Autodesk Inventor part; units mm, degrees
ref_plane "YZ Plane" through (0, 0, 0) normal (1, 0, 0) x (0, 1, 0)
ref_plane "XZ Plane" through (0, 0, 0) normal (0, 1, 0) x (-1, 0, 0)
ref_plane "XY Plane" through (0, 0, 0) normal (0, 0, 1) x (1, 0, 0)
sketch "Sketch1" plane through (0, 0, 0) normal (0, 1, 0) x (-1, 0, 0)
  line L0 (-4, 0) -> (-4, 12.7)
  line L1 (-4, 12.7) -> (-5.1, 12.7)
  line L2 (-4, 0) -> (-5.1, 0)
  line L3 (-5.1, 12.7) -> (-5.1, 8.7)
  line L4 (-5.1, 8.7) -> (-4.6, 8.7)
  line L5 (-4.6, 8.7) -> (-4.6, 7.7)
  line L6 (-4.6, 7.7) -> (-5.1, 7.7)
  line L7 (-5.1, 0) -> (-5.1, 7.7)
  line L8 (-5.1, 8.7) -> (-5.1, 12.7)
  line L9 (0, -2.54) -> (0, 15.24)
  point P0 (0, 0)
  dimension "d0" = 5.1
  dimension "d1" = 12.7
  dimension "d2" = 4
  dimension "d3" = 4
  dimension "d4" = 0.5
  dimension "d5" = 1
revolve "Revolution1" add sketch "Sketch1" angle 360 about axis through (0, 0, -10) along (0, 0, 1)
thread "Thread1"
properties part number "M8-HEATINSERT"
Check sheet for the modelled part. Datum: model origin and axes. Units: mm. A direction names the side the tool comes from. Coordinates: 2 decimals unless noted, no trailing zeros. Loops run counter-clockwise (first coordinate to the right, second up) from the corner with the lowest first, then second, coordinate; pieces in that order, holes last.
1) Sectioned sample at A-A (x = 0). Record the boundary of the cut face in (y, z).
2) Release check for a two-part mould opening along Z. For faces 3 (the face through (-3, -3, 0)), 4 (the face through (-0.867, -3.905, 6.439)), 5 (the face through (-1.2, 4.6, 7.7)) record: released by +Z, released by -Z, zero draft, split by the parting line, or undercut.
3) Sectioned sample at C-C (z = 6). Record the boundary of the cut face in (x, y), and give its area (3 significant figures).
4) Sectioned sample at B-B (y = 2). Record the boundary of the cut face in (x, z).
5) Material ranges on probe 1 along Y at (x, z) = (0, 6); probe 2 along Z at (x, y) = (-3.5, 3.5); probe 3 along Y at (x, z) = (-1, 1.75), recorded low to high.
6) Access from +Z, -Z, +X, -X, +Y, -Y to the whole of each face (thin tool, end or side, straight path). Record for faces 1 (the face through (-3, -3, 12.7)), 2 (the face through (-3.65, 2.8, 8.19)).
7) Gauge pin test, flat ends, axial feed: pin 1 (4 mm diameter, centred on x = -2.5, z = 9, fed in from -Y); pin 2 (1 mm diameter, centred on x = -1.5, z = 2, fed in from -Y); pin 3 (4 mm diameter, centred on y = 3.5, z = 3.5, fed in from -X). Record the tip position at first contact, or that the pin passes through.
Check sheet entries:
1. outline: (-5.1, 0) - (-4, 0) - (-4, 12.7) - (-5.1, 12.7) - (-5.1, 8.7) - (-4.6, 8.7) - (-4.6, 7.7) - (-5.1, 7.7) - close; (4, 0) - (5.1, 0) - (5.1, 7.7) - (4.6, 7.7) - (4.6, 8.7) - (5.1, 8.7) - (5.1, 12.7) - (4, 12.7) - close
2. face 3: released by -Z
2. face 4: zero draft
2. face 5: undercut
3. outline: circle Ø10.2 at (0, 0); hole circle Ø8 at (0, 0)
3. area: 31.4 mm2
4. outline: (-4.69, 0) - (-3.46, 0) - (-3.46, 12.7) - (-4.69, 12.7) - (-4.69, 8.7) - (-4.14, 8.7) - (-4.14, 7.7) - (-4.69, 7.7) - close; (3.46, 0) - (4.69, 0) - (4.69, 7.7) - (4.14, 7.7) - (4.14, 8.7) - (4.69, 8.7) - (4.69, 12.7) - (3.46, 12.7) - close
5. probe 1: y = -5.1 to -4, 4 to 5.1
5. probe 2: z = 0 to 7.7, 8.7 to 12.7
5. probe 3: y = -5 to -3.87, 3.87 to 5
6. face 1: +Z, +X, -X, +Y, -Y
6. face 2: none
7. pin 1: stops at y = -5.08
7. pin 2: stops at y = -5
7. pin 3: stops at x = -4.87
